Check sheet for the modelled part. Datum: model origin and axes. Units: mm. A direction names the side the tool comes from. Coordinates: 2 decimals unless noted, no trailing zeros. Loops run counter-clockwise (first coordinate to the right, second up) from the corner with the lowest first, then second, coordinate; pieces in that order, holes last.
from build123d import *

# Parameters (mm, degrees)
CROQUIS1_R               = 9
SALIENTE_EXTRUIR1_DEPTH  = 15
CORTAR_BARRER3_PROFILE_R = 0.75
CROQUIS150_W             = 9.005753034
CROQUIS150_H             = 1.22445073
SALIENTE_EXTRUIR2_DEPTH  = 15
NGULO_DE_SALIDA1_ANGLE   = 1
REDONDEO1_R              = 5
CORTAR_BARRER6_PROFILE_R = 0.75
CORTAR_BARRER7_PROFILE_R = 0.75


with BuildPart() as part:
    # Croquis1 → Saliente-Extruir1 (new body)
    with BuildSketch(Plane(origin=(0, 0, 0), x_dir=(1, 0, 0), z_dir=(0, 1, 0))):
        with BuildLine():
            Line((-10, -15.730529609), (-10, -35.730529609))
            ThreePointArc((-10, -35.730529609), (-5, -36.769633088), (0, -35.730529609))
            ThreePointArc((0, -35.730529609), (5, -36.769633088), (10, -35.730529609))
            Line((10, -35.730529609), (10, -15.730529609))
            Line((10, -15.730529609), (15, -15.730529609))
            Line((15, -15.730529609), (12.060158198, 1.375372328))
            ThreePointArc((12.060158198, 1.375372328), (15.474883642, -1.037768667), (17.888024636, 2.376956777))
            Line((17.888024636, 2.376956777), (14, 25))
            Line((14, 25), (9, 25))
            Line((9, 25), (3.3e-08, 25))
            Line((3.3e-08, 25), (-9, 25))
            Line((-9, 25), (-14, 25))
            Line((-14, 25), (-17.888024636, 2.376956777))
            ThreePointArc((-17.888024636, 2.376956777), (-15.474883642, -1.037768667), (-12.060158198, 1.375372328))
            Line((-12.060158198, 1.375372328), (-15, -15.730529609))
            Line((-15, -15.730529609), (-10, -15.730529609))
        make_face()
        with Locations(Location((0, 34, 0), (0, 0, 270))):
            Circle(CROQUIS1_R)
    extrude(amount=SALIENTE_EXTRUIR1_DEPTH)

    # Cortar-Barrer3: sweep along a path in Croquis128
    with BuildLine(Plane(origin=(0, 15, 0), x_dir=(1, 0, 0), z_dir=(0, 1, 0))) as cortar_barrer3_path:
        Line((0, -37.988500145), (0, -15.977369951))
    # Cortar-Barrer3 profile (on start of the path) → Cortar-Barrer3 (sweep, cut)
    with BuildSketch(Plane(origin=(0, 15, 37.988500145), x_dir=(-1, 0, 0), z_dir=(0, 0, -1))):
        Circle(CORTAR_BARRER3_PROFILE_R)
    sweep(path=cortar_barrer3_path.line, mode=Mode.SUBTRACT)

    # Croquis150 → Saliente-Extruir2 (add)
    with BuildSketch(Plane(origin=(0, 15, 0), x_dir=(1, 0, 0), z_dir=(0, 1, 0))):
        with Locations((0, 25.595207467)):
            Rectangle(CROQUIS150_W, CROQUIS150_H)
    extrude(amount=-SALIENTE_EXTRUIR2_DEPTH)

    # Ángulo de salida1
    ngulo_de_salida1_faces = [part.faces().sort_by_distance(p)[0] for p in [
        (0, 7.5, -43),
    ]]
    draft(ngulo_de_salida1_faces, Plane.ZX.offset(15), NGULO_DE_SALIDA1_ANGLE)

    # Redondeo1
    redondeo1_edges = [part.edges().sort_by_distance(p)[0] for p in [
        (14, 7.5, -25),
        (-14, 7.5, -25),
    ]]
    fillet(redondeo1_edges, radius=REDONDEO1_R)

    # Cortar-Barrer6: sweep along a path in Croquis153
    with BuildLine(Plane(origin=(0, 15, 0), x_dir=(1, 0, 0), z_dir=(0, 1, 0))) as cortar_barrer6_path:
        Line((-12.434351293, -0.801925236), (-9.476182309, 16.410616107))
    # Cortar-Barrer6 profile (on start of the path) → Cortar-Barrer6 (sweep, cut)
    with BuildSketch(Plane(origin=(-12.434351293, 15, 0.801925236), x_dir=(-0.9855511518924236, 0, -0.1693780593923461), z_dir=(0.1693780593923461, 0, -0.9855511518924236))):
        Circle(CORTAR_BARRER6_PROFILE_R)
    sweep(path=cortar_barrer6_path.line, mode=Mode.SUBTRACT)

    # Cortar-Barrer7: sweep along a path in Croquis222
    with BuildLine(Plane(origin=(0, 15, 0), x_dir=(1, 0, 0), z_dir=(0, 1, 0))) as cortar_barrer7_path:
        Line((9.476182309, 16.410616107), (12.355325185, -0.342100199))
    # Cortar-Barrer7 profile (on start of the path) → Cortar-Barrer7 (sweep, cut)
    with BuildSketch(Plane(origin=(9.476182309, 15, -16.410616107), x_dir=(0.9855511518924236, 0, -0.16937805939234624), z_dir=(0.16937805939234624, 0, 0.9855511518924236))):
        Circle(CORTAR_BARRER7_PROFILE_R)
    sweep(path=cortar_barrer7_path.line, mode=Mode.SUBTRACT)


solid = part.part
(1) Gauge pin test, flat ends, axial feed: P1, Ø2.5, axis at x = -6, y = 4, coming from the -Z side; P2, Ø1, axis at y = 7.5, z = -26, coming from the -X side; P3, Ø4, axis at x = -12, z = -31.5, coming from the +Y side; P4, Ø7.5, axis at y = 6.5, z = 24, coming from the -X side. Record the tip position at first contact, or that the pin passes through.
(2) Set-up check for faces 4 (the face through (10, 7, 26)), 5 (the face through (-7, 7, -25)), 6 (the face through (0.337, 7.395, -43.127)): record each of +Z, -Z, +X, -X, +Y, -Y from which the full face is reachable in a straight line by a thin tool's end or side.
(3) Scan lines: line 1 along Z through (x, y) = (6, 13.5); line 2 along X through (y, z) = (1.5, -31); line 3 along Z through (x, y) = (7, 9.5). Record each from-to range of solid material in increasing order.
(4) Section check B-B, the plane y = 13.5. Enter the section's corners in (x, z), plus the area to 3 significant figures.
(5) Section check A-A, the plane z = 31. Enter the section's corners in (x, y), plus the area to 3 significant figures.
(6) Section check D-D, the plane z = -19. Enter the section's corners in (x, y), plus the area to 3 significant figures.
(7) Section check C-C, the plane y = 4. Enter the section's corners in (x, z), plus the area to 3 significant figures.
(8) Draft check along X on faces 1 (the face through (15.41, 7.4, 1.05)), 2 (the face through (-10, 7, 26)), 3 (the face through (12, 7, 15.731)). Enter one of: pulls with the +X half, pulls with the -X half, needs draft (parallel to the pull), parting line crosses it, or undercut.
Determined:
1. P1: stops at z = -41.87
1. P2: stops at x = -5.21
1. P3: passes through
1. P4: stops at x = -10
2. face 4: +Z, +X, +Y, -Y
2. face 5: -X, +Y, -Y
2. face 6: +Y
3. line 1: z = -40.74 to -27.26, -25 to 36.73
3. line 2: x = -8.73 to 8.73
3. line 3: z = -39.81 to -28.19, -25 to 36.61
4. outline: (-17.89, -2.38) - (-14.71, -20.85) arc R5 ccw to (-9.79, -25) - (-4.5, -25) - (-4.5, -26.18) arc R9.03 ccw (long way) to (4.5, -26.18) - (4.5, -25) - (9.79, -25) arc R5 ccw to (14.71, -20.85) - (17.89, -2.38) arc R2.96 ccw to (12.06, -1.38) - (15, 15.73) - (10, 15.73) - (10, 35.73) arc R12.55 ccw to (0, 35.73) arc R12.55 ccw to (-10, 35.73) - (-10, 15.73) - (-15, 15.73) - (-12.06, -1.38) arc R2.96 ccw to start
4. area: 1,910 mm2
5. outline: (-10, 0) - (10, 0) - (10, 15) - (0.75, 15) arc R0.75 cw to (-0.75, 15) - (-10, 15) - close
5. area: 299 mm2
6. outline: (-15.03, 0) - (15.03, 0) - (15.03, 15) - (-15.03, 15) - close
6. area: 451 mm2
7. outline: (-17.89, -2.38) - (-14.71, -20.85) arc R5 ccw to (-9.79, -25) - (-4.5, -25) - (-4.5, -25.99) arc R9.19 ccw (long way) to (4.5, -25.99) - (4.5, -25) - (9.79, -25) arc R5 ccw to (14.71, -20.85) - (17.89, -2.38) arc R2.96 ccw to (12.06, -1.38) - (15, 15.73) - (10, 15.73) - (10, 35.73) arc R12.55 ccw to (0, 35.73) arc R12.55 ccw to (-10, 35.73) - (-10, 15.73) - (-15, 15.73) - (-12.06, -1.38) arc R2.96 ccw to start
7. area: 1,920 mm2
8. face 1: undercut
8. face 2: pulls with the -X half
8. face 3: needs draft
